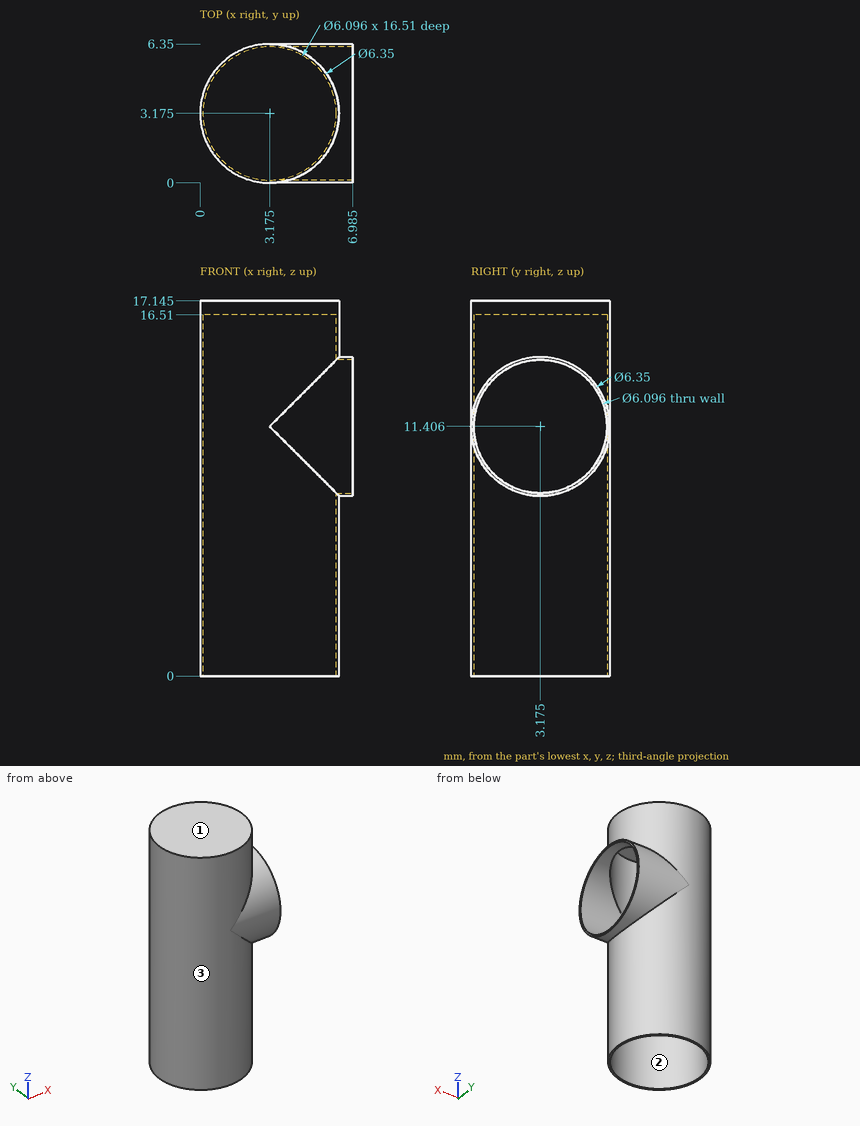
Here's the drawing with two shaded views (mm, measured from the low corner). I have some questions. Coordinates: 2 decimals unless noted, no trailing zeros. Answer as CSV lines item,"result".
Item 1: For pin 1 (1.5 mm diameter, centred on y = 1, z = 6.5, fed in from -X), with a flat end and sliding along its axis, tell me the tip position at first contact or that it passes through.
Results found:
pin 1,"x = 0.34"
Item 2: We'd pull the mould along X, two halves only. Please class the marked faces 1, 2 and 3: +X half, -X half, draft (parallel to the pull), parting line (faces both ways), or undercut.
Results found:
face 1,"draft"
face 2,"undercut"
face 3,"parting line"
Item 3: If I drill on line 1 (Z direction, x = 2, y = 2.75) (1 decimal); line 2 (X direction, y = 0.5, z = 7.5) (1 decimal); line 3 (X direction, y = 1.5, z = 14) (1 decimal), over which ranges is the centre line in solid material (lowest first)?
Results found:
line 1,"16.5 to 17.1"
line 2,"1.5 to 1.7, 4.6 to 4.9"
line 3,"0.5 to 0.6, 5.7 to 7"
